Verification items for the finished model (mm, model axes). A direction names the side the tool comes from. Give positions to 0.01 mm unless a question says otherwise; leave off trailing zeros. Loops run counter-clockwise (first coordinate to the right, second up) from the corner with the lowest first, then second, coordinate; pieces in that order, holes last. Notation, with made-up numbers: (-25, 19) -> (27, 19) arc R18 cw to (27, 35) -> close; hole circle Ø1 at (-36.75, -3). An arc over 180 degrees is marked (long way). Answer in a Markdown table with one row per item. Add a question column.
Q1. Set-up check for faces 1 (the face through (8, 46, 25)), 2 (the face through (4.06, 47.05, 17.7)): record each of +Z, -Z, +X, -X, +Y, -Y from which the full face is reachable in a straight line by a thin tool's end or side.
Q2. Section check B-B on y = 50. Enter the section's corners in (x, z).
Q3. Material ranges on probe 1 along Z at (x, y) = (4.5, 50); probe 2 along Y at (x, z) = (52.5, 22), recorded low to high.
Q4. Section check A-A on z = 35. Enter the section's corners in (x, y), and give its area (3 significant figures).
Q5. Section check C-C on z = 25. Enter the section's corners in (x, y), and give its area (3 significant figures).
Q6. Gauge pin test, flat ends, axial feed: P1, Ø13, axis at y = 50, z = 15, coming from the -X side; P2, Ø7, axis at y = 50, z = 35, coming from the -X side; P3, Ø10, axis at y = 35.5, z = 8, coming from the +X side; P4, Ø4, axis at x = 38, z = 32, coming from the +Y side. Record the tip position at first contact, or that the pin passes through.
Q7. Release check for a two-part mould opening along Y. For faces 3 (the face through (4.056, 49.479, 38.966)), 4 (the face through (7, 21, 0)), 5 (the face through (2.85, 3.01, 25.35)) record: pulls with the +Y half, pulls with the -Y half, needs draft (parallel to the pull), parting line crosses it, or undercut.
Q8. Section check D-D on x = 46.5. Enter the section's corners in (y, z).
```python
from build123d import *

# Parameters (mm, degrees)
F1_DEPTH = 50
F2_R     = 10
F3_R     = 4
F4_DEPTH = 8.001


with BuildPart() as f1:
    # F0 (on Top) → F1 (new body)
    with BuildSketch(Plane.XY):
        Polygon((8, 75), (0, 75), (0, 0), (75, 0), (75, 8), (8, 8), align=None)
    extrude(amount=F1_DEPTH)

    # F2
    f2_edges = [f1.edges().sort_by_distance(p)[0] for p in [
        (8, 8, 25),
        (0, 0, 25),
    ]]
    fillet(f2_edges, radius=F2_R)

    # F3 (on face) → F4 (cut, through all)
    with BuildSketch(Plane.YZ.offset(8)):
        with Locations((50, 35)):
            Circle(F3_R)
        with Locations((50, 15)):
            Circle(F3_R)
    extrude(amount=-F4_DEPTH, mode=Mode.SUBTRACT)


solid = f1.part
```
Taken from the geometry:
| question | item | result |
|---|---|---|
| 1 | face 1 | +Z, -Z, +X, +Y |
| 1 | face 2 | +X, -X |
| 2 | outline | (0, 0) -> (8, 0) -> (8, 11) -> (0, 11) -> close; (0, 19) -> (8, 19) -> (8, 31) -> (0, 31) -> close; (0, 39) -> (8, 39) -> (8, 50) -> (0, 50) -> close |
| 3 | probe 1 | z = 0 to 11, 19 to 31, 39 to 50 |
| 3 | probe 2 | y = 0 to 8 |
| 4 | outline | (0, 10) arc R10 ccw to (10, 0) -> (75, 0) -> (75, 8) -> (18, 8) arc R10 cw to (8, 18) -> (8, 46) -> (0, 46) -> close; (0, 54) -> (8, 54) -> (8, 75) -> (0, 75) -> close |
| 4 | area | 1,070 mm² |
| 5 | outline | (0, 10) arc R10 ccw to (10, 0) -> (75, 0) -> (75, 8) -> (18, 8) arc R10 cw to (8, 18) -> (8, 75) -> (0, 75) -> close |
| 5 | area | 1,140 mm² |
| 6 | P1 | stops at x = 0 |
| 6 | P2 | passes through |
| 6 | P3 | stops at x = 8 |
| 6 | P4 | stops at y = 8 |
| 7 | face 3 | undercut |
| 7 | face 4 | needs draft |
| 7 | face 5 | pulls with the -Y half |
| 8 | outline | (0, 0) -> (8, 0) -> (8, 50) -> (0, 50) -> close |
